from build123d import *

# Parameters (mm, degrees)
F1_DEPTH = 50.8


with BuildPart() as f1:
    # F0 (on Top) → F1 (new body)
    with BuildSketch(Plane.XY):
        with BuildLine():
            ThreePointArc((-28.628483, 23.446609), (-21.950553, 32.396332), (-19.582599, 43.308942))
            ThreePointArc((-19.582599, 43.308942), (-34.999107, 67.270107), (-63.194952, 63.171275))
            Line((-63.194952, 63.171275), (-54.316911, 52.968404))
            Line((-54.316911, 52.968404), (-52.872185, 51.308089))
            Line((-52.872185, 51.308089), (-38.250614, 34.504607))
            Line((-38.250614, 34.504607), (-28.628483, 23.446609))
        make_face()
        with BuildLine():
            Line((-54.316911, 52.968404), (-71.672229, 37.866652))
            ThreePointArc((-71.672229, 37.866652), (-66.188404, 26.513751), (-56.054994, 19.012103))
            Line((-56.054994, 19.012103), (-38.250614, 34.504607))
            Line((-38.250614, 34.504607), (-52.872185, 51.308089))
            Line((-52.872185, 51.308089), (-54.316911, 52.968404))
        make_face()
        with BuildLine():
            Line((-54.316911, 52.968404), (-63.194952, 63.171275))
            ThreePointArc((-63.194952, 63.171275), (-70.877134, 51.672582), (-71.672229, 37.866652))
            Line((-71.672229, 37.866652), (-54.316911, 52.968404))
        make_face()
        with BuildLine():
            ThreePointArc((-56.054994, 19.012103), (-41.709223, 17.317376), (-28.628483, 23.446609))
            Line((-28.628483, 23.446609), (-38.250614, 34.504607))
            Line((-38.250614, 34.504607), (-56.054994, 19.012103))
        make_face()
    extrude(amount=F1_DEPTH)


solid = f1.part
The listing builds one solid part. Answer for the finished solid, in the listing's coordinates (mm). Coordinates: 2 decimals unless noted, no trailing zeros. Write each loop counter-clockwise with the first axis right and the second up, starting at its lowest first coordinate (ties: lowest second). Pieces come first, ordered by that corner, then holes. Notation, with made-up numbers: M 15,18.5 L 56,18.5 A30 ccw 56,41.5 Z; hole C 56,11 d4. An arc over 180 degrees is marked long. Put each result on its own line as item: value. Start each with the question number.
1. A cutting plane is placed at C-C on y = 30.5. Write down the section's boundary in (x, z).
2. Consider line 1 (Y direction, x = -45, z = 42); line 2 (X direction, y = 24, z = 5.5); line 3 (X direction, y = 25, z = 34). Determine where each line is inside the solid, lowest interval first. Write a range as from..to.
3. A cutting plane is placed at A-A on z = 22. Write down the section's boundary in (x, y) (3 decimals).
4. Flat-ended cylindrical pins translate along their axes: P1, Ø6, axis at y = 57, z = 15, coming from the +X side; P2, Ø2, axis at y = 31, z = 26.5, coming from the +X side; P3, Ø6, axis at x = -55.5, z = 42, coming from the -Y side. Find the tip coordinate at first contact, or state that the pin passes through.
5. A cutting plane is placed at B-B on x = -27.5. Write down the section's boundary in (y, z).
Resolved:
1. outline: M -68.92,0 L -22.91,0 L -22.91,50.8 L -68.92,50.8 Z
2. line 1: y = 17..69.62
2. line 2: x = -63.81..-28.01
2. line 3: x = -64.83..-26.99
3. outline: M -71.672,37.867 A26.329 ccw -56.055,19.012 A26.329 ccw -28.628,23.447 A26.329 ccw -19.583,43.309 A26.329 ccw -63.195,63.171 A26.329 ccw Z
4. P1: stops at x = -21.85
4. P2: stops at x = -22.14
4. P3: stops at y = 17.82
5. outline: M 24.49,0 L 62.13,0 L 62.13,50.8 L 24.49,50.8 Z
